from build123d import *

# Parameters (mm, degrees)
F0_W        = 35
F0_H        = 35
F1_DEPTH    = 43
F2_R        = 5.35
F3_DEPTH    = 21
F4_R        = 5.35
F5_DEPTH    = 21
F6_R        = 5.35
F7_DEPTH    = 21
F8_W        = 20
F8_H        = 20
F9_DEPTH    = 43.001
F10_R       = 5.35
F11_DEPTH   = 21
F12_SIZE2   = 20
F12_SIZE    = 28
F12_2_SIZE2 = 20
F12_2_SIZE  = 28
F13_R       = 5
F14_R       = 3


with BuildPart() as f1:
    # F0 (on Top) → F1 (new body)
    with BuildSketch(Plane.XY):
        with Locations((17.5, -17.5)):
            Rectangle(F0_W, F0_H)
    extrude(amount=F1_DEPTH)

    # F2 (on face) → F3 (cut)
    with BuildSketch(Plane.XZ.offset(35)):
        with Locations((7.35, 7.35)):
            Circle(F2_R)
    extrude(amount=-F3_DEPTH, mode=Mode.SUBTRACT)

    # F4 (on face) → F5 (cut)
    with BuildSketch(Plane.YZ.offset(35)):
        with Locations((-7.35, 7.35)):
            Circle(F4_R)
    extrude(amount=-F5_DEPTH, mode=Mode.SUBTRACT)

    # F6 (on face) → F7 (cut)
    with BuildSketch(Plane.XY.offset(43)):
        with Locations((7.35, -7.35)):
            Circle(F6_R)
    extrude(amount=-F7_DEPTH, mode=Mode.SUBTRACT)

    # F8 (on face) → F9 (cut, through all)
    with BuildSketch(Plane.XY.offset(43)):
        with Locations((25, -25)):
            Rectangle(F8_W, F8_H)
    extrude(amount=-F9_DEPTH, mode=Mode.SUBTRACT)

    # F10 (on face) → F11 (cut)
    with BuildSketch(Plane(origin=(0, 0, 0), x_dir=(1, 0, 0), z_dir=(0, 0, -1))):
        with Locations((7.35, 7.35)):
            Circle(F10_R)
    extrude(amount=-F11_DEPTH, mode=Mode.SUBTRACT)

    # F12
    f12_edges = [f1.edges().sort_by_distance(p)[0] for p in [
        (35, -7.5, 43),
    ]]
    f12_side = f1.faces().sort_by_distance((35, -7.524299, 23.792232))[0]
    chamfer(f12_edges, length=F12_SIZE, length2=F12_SIZE2, reference=f12_side)

    # F12#2
    f12_2_edges = [f1.edges().sort_by_distance(p)[0] for p in [
        (7.5, -35, 43),
    ]]
    f12_2_side = f1.faces().sort_by_distance((7.524299, -35, 23.792232))[0]
    chamfer(f12_2_edges, length=F12_2_SIZE, length2=F12_2_SIZE2, reference=f12_2_side)

    # F13
    f13_edges = [f1.edges().sort_by_distance(p)[0] for p in [
        (0, 0, 21.5),
    ]]
    fillet(f13_edges, radius=F13_R)

    # F14
    f14_edges = [f1.edges().sort_by_distance(p)[0] for p in [
        (0, -25, 29),
        (25, 0, 29),
    ]]
    fillet(f14_edges, radius=F14_R)


solid = f1.part
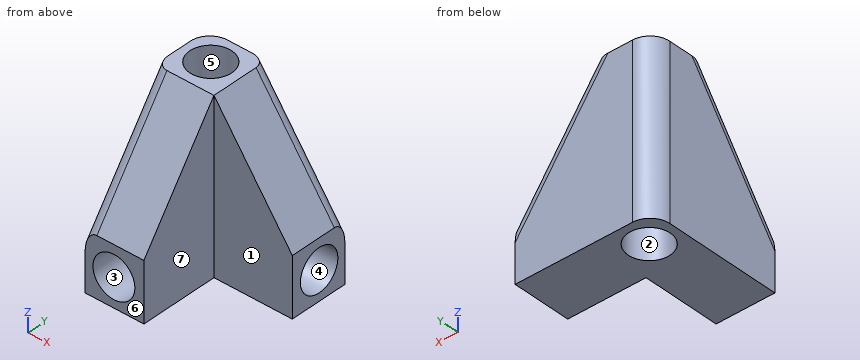
Can you work these out from the model? Positions are in its coordinate system, mm. Face numbers are marked on the shaded views. A direction names the side the tool comes from. Coordinates: 2 decimals unless noted, no trailing zeros. Loops run counter-clockwise (first coordinate to the right, second up) from the corner with the lowest first, then second, coordinate; pieces in that order, holes last. Notation, with made-up numbers: M 20,26 L 50,26 A31 cw 50,60 Z; hole C 72,87 d4. An arc over 180 degrees is marked long. Answer as CSV lines item,"result". Start each with the question number.
1. Suppose I cut it at C-C, the plane y = -7.35. List the corners of the cut face in (x, z) for me, plus the area to 3 significant figures.
2. For the marked faces 1, 2 and 3, which set-ups out of +Z, -Z, +X, -X, +Y, -Y let a thin tool reach every point of the face, with its end or its side?
3. Suppose I cut it at A-A, the plane z = 7.35. List the corners of the cut face in (x, y) for me.
4. For pin 1 Ø2 at (x, y) = (13.5, -18) entering from +Z; pin 2 Ø3 at (y, z) = (-8, 9) entering from +X; pin 3 Ø12 at (x, y) = (4.5, -26) entering from +Z, each with a flat end and sliding along its axis, tell me the tip position at first contact or that it passes through.
5. Thinking about a two-plate mould opening in Y: for the marked faces 4, 5, 6 and 7, which applies, +Y half, -Y half, draft (parallel to the pull), parting line (faces both ways), or undercut?
6. Suppose I cut it at B-B, the plane x = 7.35. List the corners of the cut face in (y, z) for me, plus the area to 3 significant figures.
7. If I drill on probe 1 along Y at (x, z) = (18, 7); probe 2 along X at (y, z) = (-29.5, 18); probe 3 along Y at (x, z) = (28.5, 9.5), over which ranges is the centre line in solid material (lowest first)? Write a range as [from, to].
Output:
1,outline,"M 0,0 L 2,0 L 2,21 L 12.7,21 L 12.7,0 L 35,0 L 35,2 L 14,2 L 14,12.7 L 35,12.7 L 35,15 L 15,43 L 12.7,43 L 12.7,22 L 2,22 L 2,43 L 0,43 Z"
1,area,"551 mm^2"
2,face 1,"+Z, -Z, +X, -Y"
2,face 2,"-Z"
2,face 3,"-Y"
3,outline,"M 0,-35 L 2,-35 L 2,-14 L 12.7,-14 L 12.7,-35 L 15,-35 L 15,-15 L 35,-15 L 35,-12.7 L 14,-12.7 L 14,-2 L 35,-2 L 35,0 L 5,0 A5 ccw 0,-5 Z; hole C 7.35,-7.35 d10.7"
4,pin 1,"stops at z = 40.2"
4,pin 2,"stops at x = 14"
4,pin 3,"stops at z = 36"
5,face 4,"undercut"
5,face 5,"undercut"
5,face 6,"-Y half"
5,face 7,"draft"
6,outline,"M -35,0 L -12.7,0 L -12.7,21 L -2,21 L -2,0 L 0,0 L 0,43 L -2,43 L -2,22 L -12.7,22 L -12.7,43 L -15,43 L -35,15 L -35,12.7 L -14,12.7 L -14,2 L -35,2 Z"
6,area,"551 mm^2"
7,probe 1,"y = [-15, -12.69], [-2.01, 0]"
7,probe 2,"x = [0.01, 15]"
7,probe 3,"y = [-15, -12.25], [-2.45, 0]"
